from build123d import *

# Parameters (mm, degrees)
SKETCH1_R           = 115
SKETCH1_R_2         = 65
SKETCH1_R_3         = 6.5
SKETCH1_R_4         = 2
BOSS_EXTRUDE1_DEPTH = 15
SKETCH2_R           = 65
BOSS_EXTRUDE2_DEPTH = 5
SKETCH4_R           = 2
CUT_EXTRUDE1_DEPTH  = 5


with BuildPart() as part:
    # Sketch1 → Boss-Extrude1 (new body)
    with BuildSketch(Plane(origin=(0, 0, 0), x_dir=(1, 0, 0), z_dir=(0, 1, 0))):
        Circle(SKETCH1_R)
        Circle(SKETCH1_R_2, mode=Mode.SUBTRACT)
        with Locations((50, 86.602540378)):
            Circle(SKETCH1_R_3, mode=Mode.SUBTRACT)
        with Locations((100, 0)):
            Circle(SKETCH1_R_3, mode=Mode.SUBTRACT)
        with Locations((50, -86.602540378)):
            Circle(SKETCH1_R_3, mode=Mode.SUBTRACT)
        with Locations((-50, -86.602540378)):
            Circle(SKETCH1_R_3, mode=Mode.SUBTRACT)
        with Locations((-100, 0)):
            Circle(SKETCH1_R_3, mode=Mode.SUBTRACT)
        with Locations((-50, 86.602540378)):
            Circle(SKETCH1_R_3, mode=Mode.SUBTRACT)
        with Locations((-25.715157224, 75.75441036)):
            Circle(SKETCH1_R_4, mode=Mode.SUBTRACT)
        with Locations((35.383095218, 71.749819323)):
            Circle(SKETCH1_R_4, mode=Mode.SUBTRACT)
        with Locations((75.75441036, 25.715157224)):
            Circle(SKETCH1_R_4, mode=Mode.SUBTRACT)
        with Locations((71.749819323, -35.383095218)):
            Circle(SKETCH1_R_4, mode=Mode.SUBTRACT)
        with Locations((25.715157224, -75.75441036)):
            Circle(SKETCH1_R_4, mode=Mode.SUBTRACT)
        with Locations((-35.383095218, -71.749819323)):
            Circle(SKETCH1_R_4, mode=Mode.SUBTRACT)
        with Locations((-75.75441036, -25.715157224)):
            Circle(SKETCH1_R_4, mode=Mode.SUBTRACT)
        with Locations((-71.749819323, 35.383095218)):
            Circle(SKETCH1_R_4, mode=Mode.SUBTRACT)
    extrude(amount=BOSS_EXTRUDE1_DEPTH)

    # Sketch2 → Boss-Extrude2 (add)
    with BuildSketch(Plane(origin=(0, 15, 0), x_dir=(1, 0, 0), z_dir=(0, 1, 0))):
        Circle(SKETCH2_R)
    extrude(amount=-BOSS_EXTRUDE2_DEPTH)

    # Sketch4 → Cut-Extrude1 (cut)
    with BuildSketch(Plane.XZ.offset(-10)):
        Circle(SKETCH4_R)
    extrude(amount=-CUT_EXTRUDE1_DEPTH, mode=Mode.SUBTRACT)


solid = part.part
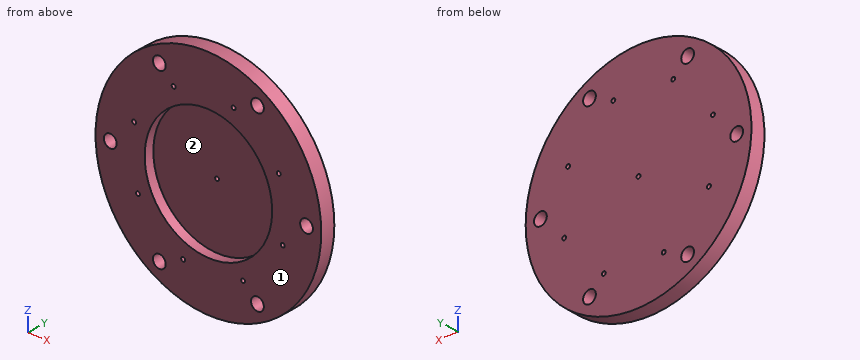
Verification items for the finished model (mm, model axes). Face numbers are marked on the shaded views. Give positions to 0.01 mm unless a question says otherwise; leave off trailing zeros. Order: outer loops, then holes, each group sorted by start corner. A loop starts at its lowest first (then second) coordinate and runs counter-clockwise, first axis right, second up. Notation, with made-up numbers: M 3,31.5 L 31,31.5 A23 ccw 31,68.5 Z; hole C -11.75,30 d7. An arc over 180 degrees is marked long. Answer as a JSON object with one key per item and string values. Group by question number.
1) Cross-section at C-C (x = -100). Enter the section's corners in (y, z), then the cut area to 3 significant figures.
2) Cross-section at D-D (x = 5). Enter the section's corners in (y, z).
3) Cross-section at B-B (x = 50). Enter the section's corners in (y, z), then the cut area to 3 significant figures.
4) Mould release check, pull along X, two halves, no side actions. Record for the marked faces 1 and 2: released by +X, released by -X, zero draft, split by the parting line, or undercut.
5) Scan lines: line 1 along Z through (x, y) = (-24, 4); line 2 along X through (y, z) = (10.5, -6); line 3 along Z through (x, y) = (50, 10.25). Record each from-to range of solid material in increasing order. Write a range as [from, to].
6) Depth check by flat-ended pin: pin 1 Ø6 at (x, y) = (41, 13.5) entering from +Z; pin 2 Ø4 at (y, z) = (11.5, -26.5) entering from -X; pin 3 Ø6 at (x, y) = (9, 3.5) entering from +Z. Enter the tip coordinate at first touch or a pass-through.
7) Cross-section at A-A (y = 5.5). Give the number of separate pieces and of enclosed holes in the cut face, then the cut area to 3 significant figures.
Result sheet:
{
 "1": {"outline": "M 0,-56.79 L 15,-56.79 L 15,-6.5 L 0,-6.5 Z; M 0,6.5 L 15,6.5 L 15,56.79 L 0,56.79 Z", "area": "1,510 mm2"},
 "2": {"outline": "M 0,-114.89 L 15,-114.89 L 15,114.89 L 0,114.89 L 0,64.81 L 10,64.81 L 10,-64.81 L 0,-64.81 Z"},
 "3": {"outline": "M 0,-103.56 L 15,-103.56 L 15,-93.1 L 0,-93.1 Z; M 0,-80.1 L 15,-80.1 L 15,80.1 L 0,80.1 L 0,41.53 L 10,41.53 L 10,-41.53 L 0,-41.53 Z; M 0,93.1 L 15,93.1 L 15,103.56 L 0,103.56 Z", "area": "1,890 mm2"},
 "4": {"face 1": "zero draft", "face 2": "undercut"},
 "5": {"line 1": "z = [-112.47, -76.78], [-74.73, -60.41], [60.41, 112.47]", "line 2": "x = [-114.84, -102.5], [-97.5, 97.5], [102.5, 114.84]", "line 3": "z = [-103.56, -93.1], [-80.1, 80.1], [93.1, 103.56]"},
 "6": {"pin 1": "stops at z = 108.54", "pin 2": "stops at x = -112.36", "pin 3": "stops at z = 114.84"},
 "7": {"separate pieces": "1", "enclosed holes": "15", "area": "27,400 mm2"}
}
